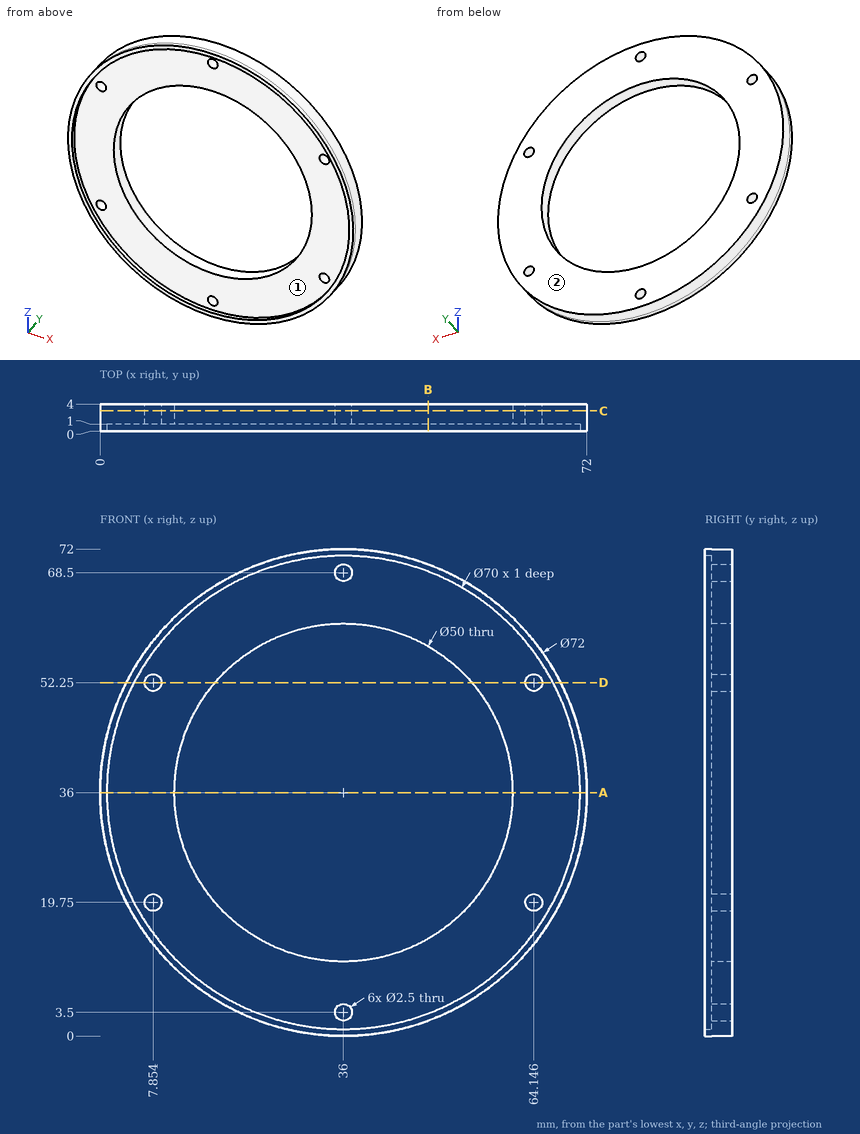
Source: three-view drawing plus pictorial views. Frame: mm from the lowest corner of the part. A direction names the side the tool comes from. Give positions to 0.01 mm unless a question says otherwise; leave off trailing zeros. Order: outer loops, then holes, each group sorted by start corner. A loop starts at its lowest first (then second) coordinate and runs counter-clockwise, first axis right, second up. Notation, with made-up numbers: M -34,83 L -23,83 A32 ccw -23,109 Z; hole C -28.75,84.25 d10. An arc over 180 degrees is marked long. Return JSON: item names as keys, results as strings.
1) Section query A-A on z = 36. Output: boundary loops of the cut face in (x, y), and give its area (3 significant figures).
Taken from the geometry:
{"outline": "M 0,0 L 1,0 L 1,1 L 11,1 L 11,4 L 0,4 Z; M 61,1 L 71,1 L 71,0 L 72,0 L 72,4 L 61,4 Z", "area": "68.0 mm2"}
2) Line query: L1, parallel to Z at x = 8, y = 2.9; L2, parallel to X at y = 3.1, z = 36; L3, parallel to X at y = 3.5, z = 19 (1 decimal). Output: solid intervals per line, ascending. Write a range as [from, to].
Taken from the geometry:
{"L1": "z = [13.37, 18.51], [20.99, 51.01], [53.49, 58.63]", "L2": "x = [0, 11], [61, 72]", "L3": "x = [4.3, 6.9], [8.9, 17.7], [54.3, 63.1], [65.1, 67.7]"}
3) Section query C-C on y = 3. Output: boundary loops of the cut face in (x, z).
Taken from the geometry:
{"outline": "C 36,36 d72; hole C 7.85,19.75 d2.5; hole C 7.85,52.25 d2.5; hole C 36,36 d50; hole C 36,3.5 d2.5; hole C 36,68.5 d2.5; hole C 64.15,19.75 d2.5; hole C 64.15,52.25 d2.5"}
4) Access query for the marked faces 1 and 2. Directions: +Z, -Z, +X, -X, +Y, -Y. A direction counts if a zero-diameter tool reaches every point of the face in a straight line with its end or side. Return the directions, or none.
Taken from the geometry:
{"face 1": "-Y", "face 2": "+Z, -Z, +X, -X, +Y"}
5) Section query D-D on z = 52.25. Output: boundary loops of the cut face in (x, y), and give its area (3 significant figures).
Taken from the geometry:
{"outline": "M 3.88,0 L 5,0 L 5,1 L 6.6,1 L 6.6,4 L 3.88,4 Z; M 9.1,1 L 17,1 L 17,4 L 9.1,4 Z; M 55,1 L 62.9,1 L 62.9,4 L 55,4 Z; M 65.4,1 L 67,1 L 67,0 L 68.12,0 L 68.12,4 L 65.4,4 Z", "area": "66.0 mm2"}
6) Contact query for flat-ended pins moving along their axis: pin 1 (4 mm diameter, centred on x = 64.15, z = 52.25, fed in from +Y); pin 2 (3 mm diameter, centred on x = 64.15, z = 19.75, fed in from -Y); pin 3 (2 mm diameter, centred on y = 3, z = 56.5, fed in from +X); pin 4 (1.5 mm diameter, centred on x = 32, y = 2, fed in from -Z). Output: stop coordinate, or through.
Taken from the geometry:
{"pin 1": "stops at y = 4", "pin 2": "stops at y = 1", "pin 3": "stops at x = 66.26", "pin 4": "stops at z = 0.15"}
7) Section query B-B on x = 48.5. Output: boundary loops of the cut face in (y, z), and give its area (3 significant figures).
Taken from the geometry:
{"outline": "M 0,2.24 L 4,2.24 L 4,14.35 L 1,14.35 L 1,3.31 L 0,3.31 Z; M 0,68.69 L 1,68.69 L 1,57.65 L 4,57.65 L 4,69.76 L 0,69.76 Z", "area": "74.8 mm2"}
